from build123d import *

# Parameters (mm, degrees)
F1_DEPTH = 25


with BuildPart() as f1:
    # F0 (on Right) → F1 (new body, symmetric)
    with BuildSketch(Plane.YZ):
        Polygon((-100, -75), (-100, -74), (-105, -74), (-105, -75), (-100.8787838708, -75), align=None)
        with BuildLine():
            Line((100, -75), (100, 75))
            ThreePointArc((100, 75), (12.7497178819, -16.6137152777), (-100, -74))
            Line((-100, -74), (-100, -75))
            Line((-100, -75), (-80, -75))
            Line((-80, -75), (-75.8787838708, -75))
            Line((-75.8787838708, -75), (-55, -75))
            Line((-55, -75), (-50.8787838708, -75))
            Line((-50.8787838708, -75), (-30, -75))
            Line((-30, -75), (-25.8787838708, -75))
            Line((-25.8787838708, -75), (-5, -75))
            Line((-5, -75), (-0.8787838708, -75))
            Line((-0.8787838708, -75), (20, -75))
            Line((20, -75), (24.1212161292, -75))
            Line((24.1212161292, -75), (45, -75))
            Line((45, -75), (49.1212161292, -75))
            Line((49.1212161292, -75), (70, -75))
            Line((70, -75), (74.1212161292, -75))
            Line((74.1212161292, -75), (95, -75))
            Line((95, -75), (99.1212161292, -75))
            Line((99.1212161292, -75), (100, -75))
        make_face()
        Polygon((129.1570463707, -75), (100, 75), (100, -75), (120, -75), (124.1212161292, -75), align=None)
        Polygon((-100.8787838708, -75), (-105, -75), (-100.8787838708, -76.5), align=None)
        Polygon((-75.8787838708, -75), (-80, -75), (-75.8787838708, -76.5), align=None)
        Polygon((-50.8787838708, -75), (-55, -75), (-50.8787838708, -76.5), align=None)
        Polygon((-25.8787838708, -75), (-30, -75), (-25.8787838708, -76.5), align=None)
        Polygon((-0.8787838708, -75), (-5, -75), (-0.8787838708, -76.5), align=None)
        Polygon((24.1212161292, -76.5), (24.1212161292, -75), (20, -75), align=None)
        Polygon((49.1212161292, -76.5), (49.1212161292, -75), (45, -75), align=None)
        Polygon((74.1212161292, -76.5), (74.1212161292, -75), (70, -75), align=None)
        Polygon((99.1212161292, -76.5), (99.1212161292, -75), (95, -75), align=None)
        Polygon((124.1212161292, -75), (120, -75), (124.1212161292, -76.5), align=None)
    extrude(amount=F1_DEPTH, both=True)


solid = f1.part
The listing builds one solid part. Answer for the finished solid, in the listing's coordinates (mm). A direction names the side the tool comes from. Round coordinates to 2 decimals unless told otherwise and drop trailing zeros. Loops run counter-clockwise (first coordinate to the right, second up) from the corner with the lowest first, then second, coordinate; pieces in that order, holes last. Notation, with made-up numbers: M 52,13.25 L 88,13.25 A9 ccw 88,21.25 Z; hole C 16,-12.75 d7. An arc over 180 degrees is marked long. Return JSON: item names as keys, results as strings.
Q1. Which of the six approach directions +Z, -Z, +X, -X, +Y, -Y give full straight-line access (tool end or side, diameter ignored) to faces 5 (the face through (0, 127, -75)), 6 (the face through (0, -16, -75)), 7 (the face through (0, -102, -74))?
Results list:
{"face 5": "-Z, +X, -X, +Y", "face 6": "-Z, +X, -X", "face 7": "+Z, +X, -X, -Y"}
Q2. Find section B-B, the plane y = 39. Determine the outline of the cut face in (x, z), plus the area to 3 significant figures.
Results list:
{"outline": "M -25,-75 L 25,-75 L 25,4.85 L -25,4.85 Z", "area": "3,990 mm2"}
Q3. Find the intervals of material crossed by line 1 along Z through (x, y) = (-3.5, 1); line 2 along Z through (x, y) = (2, -75); line 3 along Y through (x, z) = (-18, -26), in increasing order. Write a range as from..to.
Results list:
{"line 1": "z = -75..-25.02", "line 2": "z = -75..-65.25", "line 3": "y = -0.43..119.63"}
Q4. Find section C-C, the plane z = 12. Determine the outline of the cut face in (x, y).
Results list:
{"outline": "M -25,46.75 L 25,46.75 L 25,112.25 L -25,112.25 Z"}
Q5. Each of these flat-tipped pins is pushed along its axis until it touches: pin 1 Ø12 at (x, z) = (-5.5, -17.5) entering from -Y; pin 2 Ø5 at (x, y) = (16, 92) entering from -Z; pin 3 Ø16.5 at (x, y) = (10, 4.5) entering from -Z. Where does it stop, or does it pass through?
Results list:
{"pin 1": "stops at y = 3.2", "pin 2": "stops at z = -75", "pin 3": "stops at z = -76.5"}
Q6. The mould has two halves that part along Y. Classify faces 1 (the face through (25, 62, -33)), 2 (the face through (0, 84, -75)), 3 (the face through (0.35, 114.783, -1.05)), 4 (the face through (0, -41, -75)): released by +Y, released by -Y, zero draft, split by the parting line, or undercut.
Results list:
{"face 1": "zero draft", "face 2": "undercut", "face 3": "released by +Y", "face 4": "undercut"}
